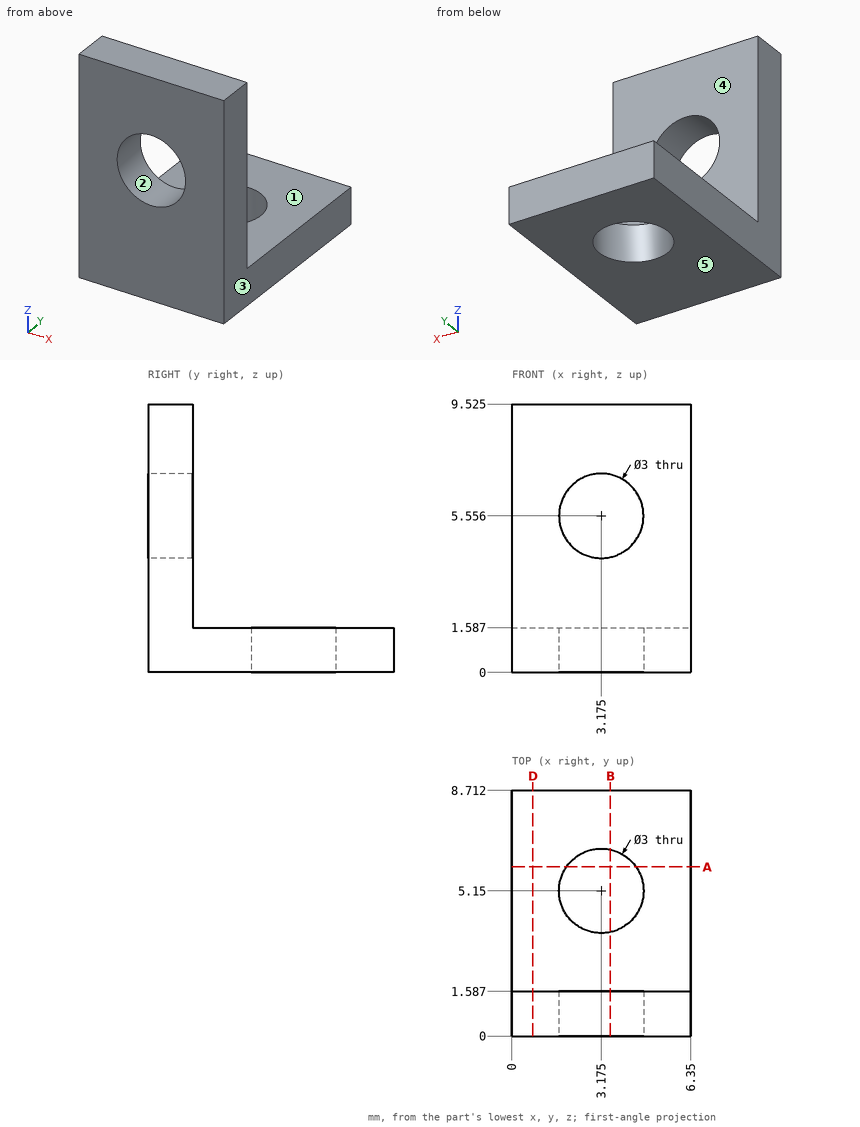
Verification items for this drawing (mm, ordinates from the low corner). A direction names the side the tool comes from. Coordinates: 2 decimals unless noted, no trailing zeros. Write each loop counter-clockwise with the first axis right and the second up, starting at its lowest first coordinate (ties: lowest second). Pieces come first, ordered by that corner, then holes. Notation, with made-up numbers: M 66,0 L 117,0 A13 ccw 117,5 Z; hole C 70,-7.5 d9. An arc over 180 degrees is marked long. One line per item, written item: value. Start each with the question number.
(1) Scan lines: line 1 along Y through (x, z) = (2, 8.75); line 2 along X through (y, z) = (6, 1.25). Record each from-to range of solid material in increasing order. Write a range as [from, to].
(2) Tool access check on the marked faces 4 and 5. Record the directions out of +Z, -Z, +X, -X, +Y, -Y that give a thin tool (end or side, any length) a straight path to the whole face; none if there is none.
(3) Sectioned sample at D-D, the plane x = 0.75. Enter the section's corners in (y, z) (1 decimal).
(4) Release check for a two-part mould opening along X. For the marked faces 1, 2 and 3 record: released by +X, released by -X, zero draft, split by the parting line, or undercut.
(5) Sectioned sample at A-A, the plane y = 6. Enter the section's corners in (x, z).
(6) Sectioned sample at B-B, the plane x = 3.5. Enter the section's corners in (y, z) (1 decimal).
(7) Depth check by flat-ended pin: pin 1 (2 mm diameter, centred on x = 1, y = 3, fed in from +Z); pin 2 (3 mm diameter, centred on x = 5.5, y = 2, fed in from -Z); pin 3 (2.5 mm diameter, centred on x = 3.18, z = 5.56, fed in from +Y); pin 4 (1.9 mm diameter, centred on x = 3, z = 5, fed in from +Y). Enter the tip coordinate at first touch or a pass-through.
Filled sheet:
1. line 1: [0, 1.59]
1. line 2: [0, 1.94], [4.41, 6.35]
2. face 4: +Z, +X, -X, +Y
2. face 5: -Z, +X, -X, +Y, -Y
3. outline: M 0,0 L 8.7,0 L 8.7,1.6 L 1.6,1.6 L 1.6,9.5 L 0,9.5 Z
4. face 1: zero draft
4. face 2: undercut
4. face 3: released by +X
5. outline: M 0,0 L 1.94,0 L 1.94,1.59 L 0,1.59 Z; M 4.41,0 L 6.35,0 L 6.35,1.59 L 4.41,1.59 Z
6. outline: M 0,0 L 3.7,0 L 3.7,1.6 L 1.6,1.6 L 1.6,4.1 L 0,4.1 Z; M 0,7 L 1.6,7 L 1.6,9.5 L 0,9.5 Z; M 6.6,0 L 8.7,0 L 8.7,1.6 L 6.6,1.6 Z
7. pin 1: z = 1.59
7. pin 2: z = 0
7. pin 3: through
7. pin 4: y = 1.59
